Could you check a few things on this drawing? It's one solid part, dimensions in mm from its lowest x, y, z. A direction names the side the tool comes from. Round coordinates to 2 decimals unless told otherwise and drop trailing zeros. Write each loop counter-clockwise with the first axis right and the second up, starting at its lowest first coordinate (ties: lowest second). Pieces come first, ordered by that corner, then holes. Notation, with made-up numbers: (32, 50.5) -> (85, 50.5) arc R36 ccw to (85, 85.5) -> close; hole circle Ø8 at (2, 52.5). An arc over 180 degrees is marked (long way). Answer in a Markdown table with one row per item.
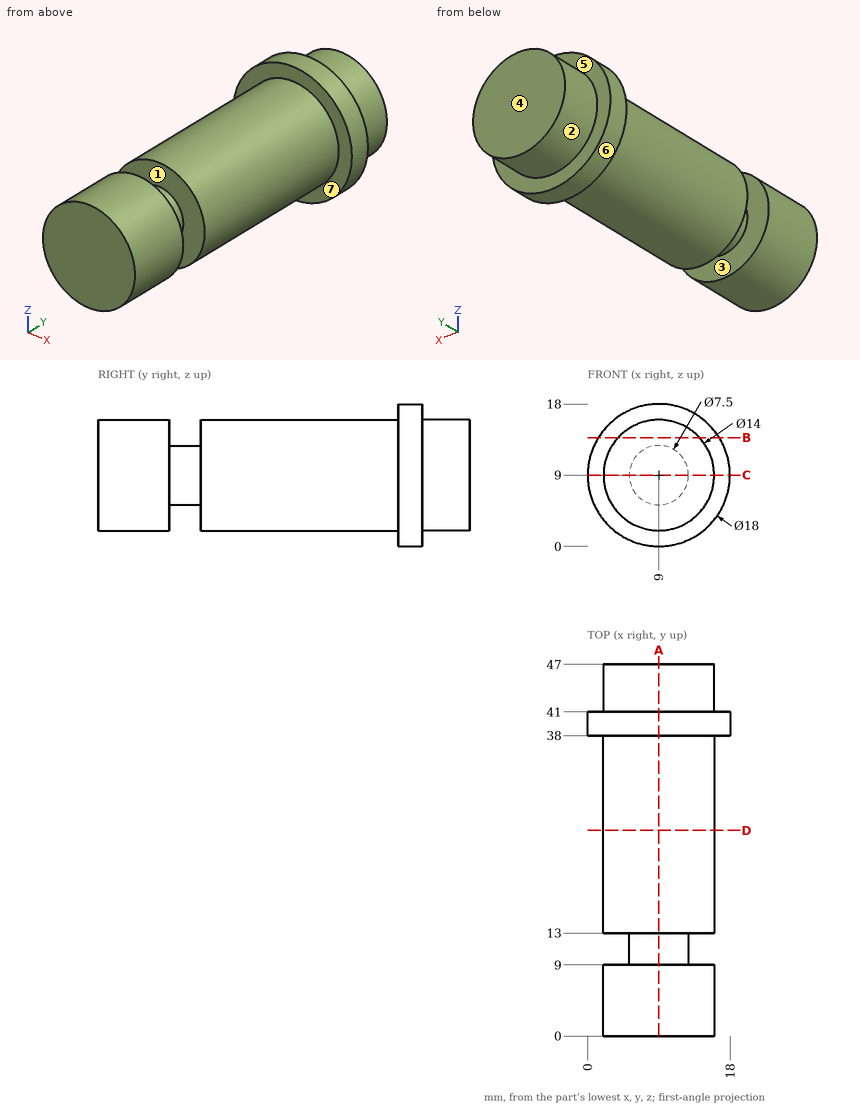
1) I want a section at A-A, the plane x = 9. List the corners of the cut face in (y, z) for me, and give its area (3 significant figures).
Response:
| item | result |
|---|---|
| outline | (0, 2) -> (9, 2) -> (9, 5.25) -> (13, 5.25) -> (13, 2) -> (38, 2) -> (38, 0) -> (41, 0) -> (41, 2) -> (47, 2) -> (47, 16) -> (41, 16) -> (41, 18) -> (38, 18) -> (38, 16) -> (13, 16) -> (13, 12.75) -> (9, 12.75) -> (9, 16) -> (0, 16) -> close |
| area | 644 mm^2 |
2) We'd pull the mould along Y, two halves only. Please class the marked faces 1, 2, 3 and 4: +Y half, -Y half, draft (parallel to the pull), parting line (faces both ways), or undercut.
Response:
| item | result |
|---|---|
| face 1 | undercut |
| face 2 | draft |
| face 3 | undercut |
| face 4 | +Y half |
3) Which directions (+Z, -Z, +X, -X, +Y, -Y) give clear straight access to the entire face, cutting with the end or side of a thin tool? Please do the marked faces 5, 6 and 7.
Response:
| item | result |
|---|---|
| face 5 | +Y |
| face 6 | +Y, -Y |
| face 7 | -Y |
4) I want a section at C-C, the plane z = 9. List the corners of the cut face in (x, y) for me, and give its area (3 significant figures).
Response:
| item | result |
|---|---|
| outline | (0, 38) -> (2, 38) -> (2, 13) -> (5.25, 13) -> (5.25, 9) -> (2, 9) -> (2, 0) -> (16, 0) -> (16, 9) -> (12.75, 9) -> (12.75, 13) -> (16, 13) -> (16, 38) -> (18, 38) -> (18, 41) -> (16, 41) -> (16, 47) -> (2, 47) -> (2, 41) -> (0, 41) -> close |
| area | 644 mm^2 |
5) For pin 1 (2 mm diameter, centred on y = 40.5, z = 13, fed in from +X); pin 2 (2 mm diameter, centred on x = 15.5, y = 21.5, fed in from +Z); pin 3 (3 mm diameter, centred on y = 8, z = 9, fed in from +X), each with a flat end and sliding along its axis, tell me the tip position at first contact or that it passes through.
Response:
| item | result |
|---|---|
| pin 1 | stops at x = 17.49 |
| pin 2 | stops at z = 13.33 |
| pin 3 | stops at x = 16 |
6) I want a section at B-B, the plane z = 13.75. List the corners of the cut face in (x, y) for me, and give its area (3 significant figures).
Response:
| item | result |
|---|---|
| outline | (1.36, 38) -> (3.86, 38) -> (3.86, 13) -> (14.14, 13) -> (14.14, 38) -> (16.64, 38) -> (16.64, 41) -> (14.14, 41) -> (14.14, 47) -> (3.86, 47) -> (3.86, 41) -> (1.36, 41) -> close; (3.86, 0) -> (14.14, 0) -> (14.14, 9) -> (3.86, 9) -> close |
| area | 457 mm^2 |
7) I need wall thicknesses on line 1 (Y direction, x = 10.25, z = 3.25); line 2 (Y direction, x = 3, z = 14); line 3 (X direction, y = 24, z = 9.25). Which ranges of each line are inside material? Lowest first, please. Write a range as [from, to].
Response:
| item | result |
|---|---|
| line 1 | y = [0, 9], [13, 47] |
| line 2 | y = [38, 41] |
| line 3 | x = [2, 16] |
8) I want a section at D-D, the plane y = 26. List the corners of the cut face in (x, z) for me.
Response:
| item | result |
|---|---|
| outline | circle Ø14 at (9, 9) |
